```python
from build123d import *

# Parameters (mm, degrees)
BOSS_EXTRUDE1_DEPTH = 5
SKETCH2_R           = 1.4
CUT_EXTRUDE1_DEPTH  = 8
SKETCH3_R           = 1.4
CUT_EXTRUDE2_DEPTH  = 6
FILLET1_R           = 2


with BuildPart() as part:
    # Sketch1 → Boss-Extrude1 (new body)
    with BuildSketch(Plane.XY):
        Polygon((-12.363085779, 11.239336475), (-6.033085779, 11.239336475), (-6.033085779, 6.489336475), (-4.698085779, 6.489336475), (-4.698085779, -5.260663525), (-13.698085779, -5.260663525), (-13.698085779, 6.489336475), (-12.363085779, 6.489336475), align=None)
        Polygon((-9.198085779, 4.489336475), (-6.198085779, 4.489336475), (-6.198085779, -3.760663525), (-12.198085779, -3.760663525), (-12.198085779, 4.489336475), align=None, mode=Mode.SUBTRACT)
    extrude(amount=BOSS_EXTRUDE1_DEPTH)

    # Sketch2 → Cut-Extrude1 (cut)
    with BuildSketch(Plane(origin=(-6.033085779, 0, 0), x_dir=(0, 0, -1), z_dir=(1, 0, 0))):
        with Locations((-2.5, 9.323502588)):
            Circle(SKETCH2_R)
    extrude(amount=-CUT_EXTRUDE1_DEPTH, mode=Mode.SUBTRACT)

    # Sketch3 → Cut-Extrude2 (cut)
    with BuildSketch(Plane.XZ.offset(5.260663525)):
        with Locations((-9.198085779, 2.5)):
            Circle(SKETCH3_R)
    extrude(amount=-CUT_EXTRUDE2_DEPTH, mode=Mode.SUBTRACT)

    # Fillet1
    fillet1_edges = [part.edges().sort_by_distance(p)[0] for p in [
        (-9.198085779, 11.239336475, 5),
        (-9.198085779, 11.239336475, 0),
    ]]
    fillet(fillet1_edges, radius=FILLET1_R)


solid = part.part
```
Work out the finished part from the listing and answer in its coordinate system (mm). A direction names the side the tool comes from. Round coordinates to 2 decimals unless told otherwise and drop trailing zeros. Loops run counter-clockwise (first coordinate to the right, second up) from the corner with the lowest first, then second, coordinate; pieces in that order, holes last.
(1) The mould has two halves that part along Z. Classify faces 1 (the cylindrical face through (-9.15, 10.67, 0.6)), 2 (the cylindrical face through (-7.905, -4.521, 1.964)), 3 (the flat face through (-12.363, 7.8, 1.9)), 4 (the cylindrical face through (-9.154, 10.504, 1.747)): pulls with the +Z half, pulls with the -Z half, needs draft (parallel to the pull), parting line crosses it, or undercut.
Computed values:
face 1: pulls with the -Z half
face 2: undercut
face 3: needs draft
face 4: undercut
(2) Find the intervals of material crossed by L1, parallel to X at y = 0, z = 4.25; L2, parallel to Y at x = -7, z = 2.6; L3, parallel to Y at x = -12.75, z = 0.7, in increasing order.
Computed values:
L1: x = -13.7 to -12.2, -6.2 to -4.7
L2: y = -5.26 to -3.76, 4.49 to 7.93, 10.72 to 11.24
L3: y = -5.26 to 6.49
(3) For faces 5 (the flat face through (-6.033, 7.8, 3)), 6 (the flat face through (-9, 4.489, 2)), 7 (the flat face through (-13, 6.489, 2)), determine the directions among +Z, -Z, +X, -X, +Y, -Y from which every point of the face is accessible in a straight line to the end or side of a thin tool.
Computed values:
face 5: +Z, -Z, +X, +Y
face 6: +Z, -Z
face 7: +Z, -Z, -X, +Y
(4) The part is cut by section C-C, the plane x = -8. Give the vertices of the cut face in (y, z), and give its area (3 significant figures).
Computed values:
outline: (-5.26, 0) - (-3.76, 0) - (-3.76, 1.78) - (-5.26, 1.78) - close; (-5.26, 3.22) - (-3.76, 3.22) - (-3.76, 5) - (-5.26, 5) - close; (4.49, 0) - (9.24, 0) arc R2 ccw to (11.24, 2) - (11.24, 3) arc R2 ccw to (9.24, 5) - (4.49, 5) - close; hole circle Ø2.8 at (9.32, 2.5)
area: 31.2 mm2
(5) The part is cut by section B-B, the plane z = 2.5. Give the vertices of the cut face in (x, y).
Computed values:
outline: (-13.7, -5.26) - (-10.6, -5.26) - (-10.6, -3.76) - (-12.2, -3.76) - (-12.2, 4.49) - (-6.2, 4.49) - (-6.2, -3.76) - (-7.8, -3.76) - (-7.8, -5.26) - (-4.7, -5.26) - (-4.7, 6.49) - (-6.03, 6.49) - (-6.03, 7.92) - (-12.36, 7.92) - (-12.36, 6.49) - (-13.7, 6.49) - close; (-12.36, 10.72) - (-6.03, 10.72) - (-6.03, 11.24) - (-12.36, 11.24) - close
(6) The part is cut by section A-A, the plane x = -12. Give the vertices of the cut face in (y, z).
Computed values:
outline: (-5.26, 0) - (-3.76, 0) - (-3.76, 5) - (-5.26, 5) - close; (4.49, 0) - (9.24, 0) arc R2 ccw to (11.24, 2) - (11.24, 3) arc R2 ccw to (9.24, 5) - (4.49, 5) - close; hole circle Ø2.8 at (9.32, 2.5)
(7) Each of these flat-tipped pins is pushed along its axis until it touches: P1, Ø1, axis at x = -10, y = 2, coming from the +Z side; P2, Ø1.5, axis at x = -8.5, z = 4, coming from the +Y side; P3, Ø2.5, axis at y = 9.5, z = 2, coming from the +X side; P4, Ø2.5, axis at y = 9, z = 2, coming from the -X side. Where does it stop, or does it pass through?
Computed values:
P1: passes through
P2: stops at y = 11.22
P3: stops at x = -6.03
P4: stops at x = -12.36
(8) The part is cut by section D-D, the plane y = -1. Give the vertices of the cut face in (x, z).
Computed values:
outline: (-13.7, 0) - (-12.2, 0) - (-12.2, 5) - (-13.7, 5) - close; (-6.2, 0) - (-4.7, 0) - (-4.7, 5) - (-6.2, 5) - close
